Check sheet for the modelled part. Datum: model origin and axes. Units: mm. A direction names the side the tool comes from. Coordinates: 2 decimals unless noted, no trailing zeros. Order: outer loops, then holes, each group sorted by start corner. A loop starts at its lowest first (then second) coordinate and runs counter-clockwise, first axis right, second up. Notation, with made-up numbers: M 77,-13.75 L 108,-13.75 A18 ccw 108,-6.75 Z; hole C 44,-14 d6. An arc over 180 degrees is marked long. Answer in a Markdown table with one row per item. Add a question column.
from build123d import *

# Parameters (mm, degrees)
F1_DEPTH = 33.274
F2_DEPTH = 25.4


with BuildPart() as f1:
    # F0 (on Right) → F1 (new body)
    with BuildSketch(Plane.YZ):
        Polygon((0, 50.9521476924), (-19.1701129079, 50.9521476924), (-19.1701129079, 23.7104035914), (-48.4297610819, 0), (-48.4297610819, -46.5127490461), (0, -46.5127490461), (48.4297610819, -46.5127490461), (48.4297610819, 0), (19.1701129079, 23.7104035914), (19.1701129079, 50.9521476924), align=None)
    extrude(amount=F1_DEPTH)

    # F2 (add): faces of the model
    f2_faces = [f1.faces().sort_by_distance(p)[0] for p in [
        (16.637, -33.7999369949, 11.8552017957),
        (16.637, -48.4297610819, -23.256374523),
        (16.637, -19.1701129079, 37.3312756419),
    ]]
    extrude(f2_faces, amount=F2_DEPTH, dir=(0, -0.6295834828, 0.7769328402))


solid = f1.part
1. Go/stop test with flat-tipped pins: pin 1 Ø3 at (x, z) = (17.5, 26) entering from -Y; pin 2 Ø3 at (x, z) = (6.5, 36) entering from +Y; pin 3 Ø4 at (x, z) = (18.5, 38) entering from -Y. Record where each tip stops, or that it passes through.
2. Section check B-B on y = -10. Enter the section's corners in (x, z).
3. Scan lines: line 1 (Z direction, x = 29, y = 9); line 2 (Y direction, x = 15.5, z = -30); line 3 (Z direction, x = 7.5, y = 29.5). Record each from-to range of solid material in increasing order.
4. Section check C-C on z = -31. Enter the section's corners in (x, y), then the cut area to 3 significant figures.
5. Set-up check for faces 1 (the flat face through (16, -35.162, 57)), 2 (the flat face through (16, 19.17, 37)), 3 (the flat face through (33.274, -10, -3)): record each of +Z, -Z, +X, -X, +Y, -Y from which the full face is reachable in a straight line by a thin tool's end or side.
6. Section check A-A on x = 21. Enter the section's corners in (y, z).
Result sheet:
| question | item | result |
|---|---|---|
| 1 | pin 1 | y = -58.54 |
| 1 | pin 2 | y = 19.17 |
| 1 | pin 3 | y = -44.35 |
| 2 | outline | M 0,-46.51 L 33.27,-46.51 L 33.27,50.95 L 0,50.95 Z |
| 3 | line 1 | -46.51 to 50.95 |
| 3 | line 2 | -61.81 to 48.43 |
| 3 | line 3 | -46.51 to 15.34 |
| 4 | outline | M 0,-61 L 33.27,-61 L 33.27,48.43 L 0,48.43 Z |
| 4 | area | 3,640 mm^2 |
| 5 | face 1 | +Z, +X, -X, -Y |
| 5 | face 2 | +Z, +X, -X, +Y |
| 5 | face 3 | +Z, -Z, +X, +Y, -Y |
| 6 | outline | M -64.42,-26.78 L -48.43,-46.51 L 48.43,-46.51 L 48.43,0 L 19.17,23.71 L 19.17,50.95 L -19.17,50.95 L -35.16,70.69 L -35.16,43.44 L -64.42,19.73 Z |
